Print and shaded views of the part. All mm, measured from the part's lowest x, y and z. Coordinates: 2 decimals unless noted, no trailing zeros. One line per item, written item: value.
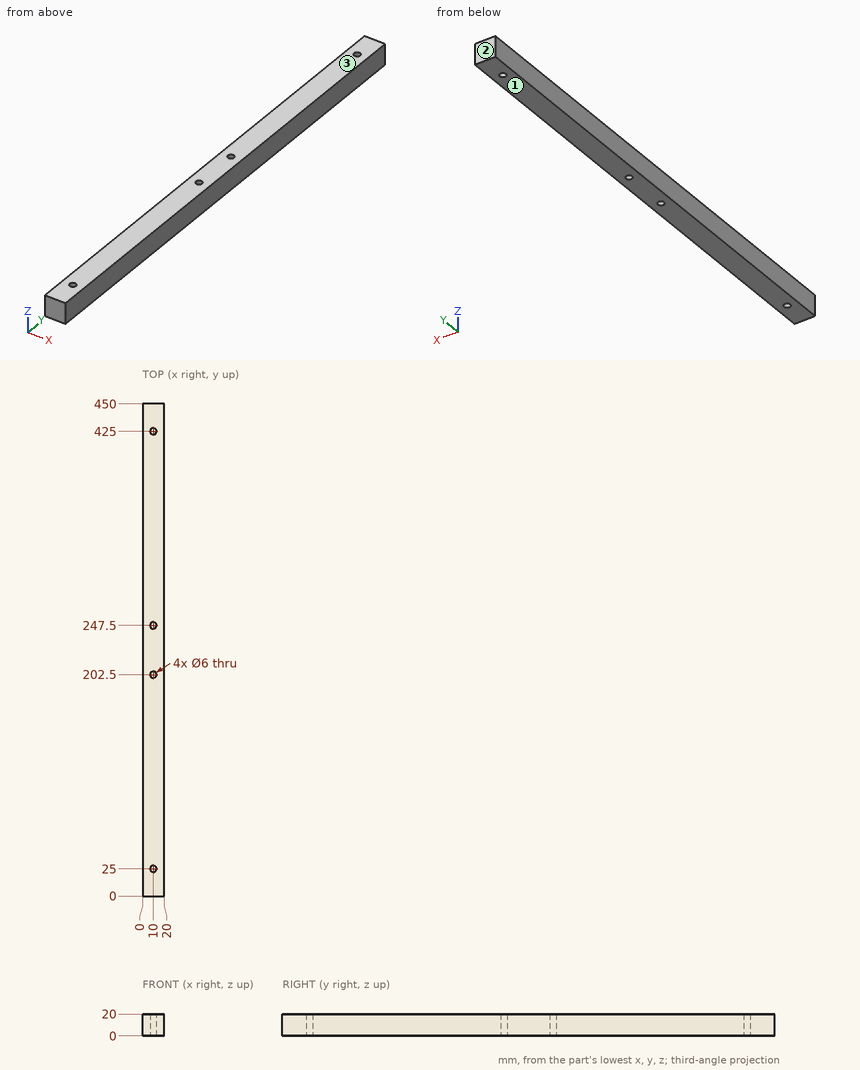
Q1. Drill centre lines: line 1 along Y through (x, z) = (10, 15.25); line 2 along X through (y, z) = (425, 8); line 3 along X through (y, z) = (250, 10). Where is each one in solid material? Low to high.
Recorded:
line 1: y = 0 to 22, 28 to 199.5, 205.5 to 244.5, 250.5 to 422, 428 to 450
line 2: x = 0 to 7, 13 to 20
line 3: x = 0 to 8.34, 11.66 to 20
Q2. Mould opens along Z. For the marked faces 1, 2 and 3 say: released by +Z, released by -Z, zero draft, split by the parting line, or undercut.
Recorded:
face 1: released by -Z
face 2: zero draft
face 3: released by +Z
Q3. Pin check, flat tip, straight feed: pin 1 Ø5.5 at (x, y) = (10, 202.5) entering from -Z. Stop position of the tip, or through.
Recorded:
pin 1: passes through
